Work out the finished part from the listing and answer in its coordinate system (mm). Round coordinates to 2 decimals unless told otherwise and drop trailing zeros. Loops run counter-clockwise (first coordinate to the right, second up) from the corner with the lowest first, then second, coordinate; pieces in that order, holes last.
```python
from build123d import *

# Parameters (mm, degrees)
F0_W     = 88.9
F0_H     = 127
F1_DEPTH = 203.2
F2_R     = 31.75
F3_R     = 31.75


with BuildPart() as f1:
    # F0 (on Right) → F1 (new body)
    with BuildSketch(Plane.YZ):
        with Locations((44.45, 63.5)):
            Rectangle(F0_W, F0_H)
    extrude(amount=F1_DEPTH)

    # F2
    f2_edges = [f1.edges().sort_by_distance(p)[0] for p in [
        (101.6, 88.9, 127),
    ]]
    fillet(f2_edges, radius=F2_R)

    # F3
    f3_edges = [f1.edges().sort_by_distance(p)[0] for p in [
        (101.6, 88.9, 0),
    ]]
    fillet(f3_edges, radius=F3_R)


solid = f1.part
```
1. Find section A-A (x = 156.5). Write down the section's boundary in (y, z), then the cut area to 3 significant figures.
Answer key:
outline: (0, 0) - (57.15, 0) arc R31.75 ccw to (88.9, 31.75) - (88.9, 95.25) arc R31.75 ccw to (57.15, 127) - (0, 127) - close
area: 10,900 mm2
2. Find section C-C (y = 78). Write down the section's boundary in (x, z).
Answer key:
outline: (0, 7.81) - (203.2, 7.81) - (203.2, 119.19) - (0, 119.19) - close
3. Find section B-B (z = 119). Write down the section's boundary in (x, y), then the cut area to 3 significant figures.
Answer key:
outline: (0, 0) - (203.2, 0) - (203.2, 78.22) - (0, 78.22) - close
area: 15,900 mm2
4. Consider probe 1 along Z at (x, y) = (77, 61.5); probe 2 along Y at (x, z) = (36, 6); probe 3 along Y at (x, z) = (145.5, 102.5). Determine where each line is inside the solid, lowest interval first.
Answer key:
probe 1: z = 0.3 to 126.7
probe 2: y = 0 to 75.72
probe 3: y = 0 to 88.06
5. Given pin 1 (1 mm diameter, centred on x = 72, z = 14.5, fed in from -Y); pin 2 (1.5 mm diameter, centred on x = 108, z = 16, fed in from +Y), each flat-ended and moving along its own axis, determine where each tip first touches the part or whether it passes through.
Answer key:
pin 1: stops at y = 0
pin 2: stops at y = 85.13
